Build history of the part. All positions in model axes, mm. Face numbers are marked on the shaded views. A direction names the side the tool comes from. Give positions to 0.01 mm unless a question says otherwise; leave off trailing zeros. Order: outer loops, then holes, each group sorted by start corner. A loop starts at its lowest first (then second) coordinate and runs counter-clockwise, first axis right, second up. Notation, with made-up numbers: (31.5, 89) - (79.5, 89) arc R26 ccw to (79.5, 117) - close; hole circle Ø5 at (58, 11). An arc over 180 degrees is marked (long way). Write each question's results on one line, items separated by ' | '. Start each with the question number.
1) Drill centre lines: line 1 along Y through (x, z) = (0, 2.4); line 2 along Z through (x, y) = (3, -6); line 3 along X through (y, z) = (-2.75, 16.5). Where is each one in solid material? Low to high. Write a range as from..to.
2) Cut at C-C on y = 0. List the corners of the cut face in (x, z).
3) Cut at D-D on y = 7.5. List the corners of the cut face in (x, z), plus the area to 3 significant figures.
4) Tool access for the marked faces 5 and 6: list every direction of +Z, -Z, +X, -X, +Y, -Y with a clear straight run to the whole face (end or side of a thin tool).
5) Drop flat-ended pins along their axis: pin 1 Ø12 at (y, z) = (-7, 11) entering from -X; pin 2 Ø10 at (x, y) = (0, 0) entering from -Z; pin 3 Ø1 at (y, z) = (-3.5, 5.5) entering from -X; pin 4 Ø6 at (y, z) = (0, 24) entering from -X. Give the stop position or say it passes through.
6) Two-plate mould, pull along Z, no slides. Class the marked faces 1, 2, 3 and 4: +Z half, -Z half, draft (parallel to the pull), parting line (faces both ways), or undercut.
7) Cut at A-A on x = -3. List the corners of the cut face in (y, z).
8) Cut at B-B on z = 24. List the corners of the cut face in (x, y).
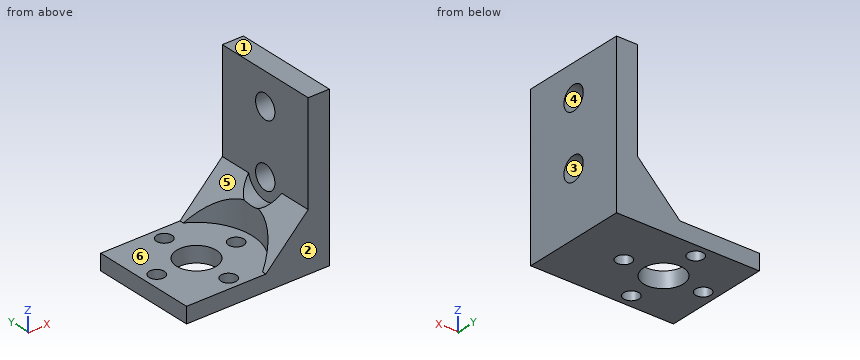
from build123d import *

# Parameters (mm, degrees)
SKETCH_1_W                   = 20
SKETCH_1_H                   = 20
EXTRUDE_1_DEPTH              = 3
SKETCH_8_W                   = 3
SKETCH_8_H                   = 20
EXTRUDE_3_DEPTH              = 3
SKETCH_2_R                   = 3.75
CUT_EXTRUDE_1_DEPTH          = 17.673332001
SKETCH_3_W                   = 4
SKETCH_3_H                   = 20
EXTRUDE_2_DEPTH              = 30
CHAMFER_1_SIZE               = 8
SKETCH_9_R                   = 10.5
CUT_EXTRUDE_2_DEPTH          = 27
HOLE_WIZARD_M4_1_D           = 4.5
HOLE_WIZARD_M4_1_CBORE_D     = 8
HOLE_WIZARD_M4_1_CBORE_DEPTH = 23
HOLE_WIZARD_M2_5_1_D         = 2.9


with BuildPart() as part:
    # 草圖1 → 填料-伸長1 (new body)
    with BuildSketch(Plane.XY):
        Rectangle(SKETCH_1_W, SKETCH_1_H)
    extrude(amount=EXTRUDE_1_DEPTH)

    # 草圖8 → 填料-伸長3 (add)
    with BuildSketch(Plane(origin=(10, 0, 0), x_dir=(0, 0, -1), z_dir=(1, 0, 0))):
        with Locations((-1.5, 0)):
            Rectangle(SKETCH_8_W, SKETCH_8_H)
    extrude(amount=EXTRUDE_3_DEPTH)

    # 草圖2 → 除料-伸長1 (cut, through all)
    with BuildSketch(Plane.XY.offset(3)):
        Circle(SKETCH_2_R)
    extrude(amount=-CUT_EXTRUDE_1_DEPTH, mode=Mode.SUBTRACT)

    # 草圖3 → 填料-伸長2 (add)
    with BuildSketch(Plane(origin=(0, 0, 0), x_dir=(-1, 0, 0), z_dir=(0, 0, -1))):
        with Locations((-15, 0)):
            Rectangle(SKETCH_3_W, SKETCH_3_H)
    extrude(amount=-EXTRUDE_2_DEPTH)

    # 導角1
    chamfer_1_edges = [part.edges().sort_by_distance(p)[0] for p in [
        (13, 0, 3),
    ]]
    chamfer(chamfer_1_edges, length=CHAMFER_1_SIZE)

    # 草圖9 → 除料-伸長2 (cut)
    with BuildSketch(Plane.XY.offset(30)):
        Circle(SKETCH_9_R)
    extrude(amount=-CUT_EXTRUDE_2_DEPTH, mode=Mode.SUBTRACT)

    # M4 凹頭蓋螺釘的柱孔1 (through all)
    with Locations(Plane.ZY.offset(10)):
        with Locations((24, 0), (12, 0)):
            CounterBoreHole(HOLE_WIZARD_M4_1_D / 2, HOLE_WIZARD_M4_1_CBORE_D / 2, HOLE_WIZARD_M4_1_CBORE_DEPTH)

    # M2.5 餘隙孔1 (through all)
    with Locations(Plane(origin=(0, 0, 0), x_dir=(-1, 0, 0), z_dir=(0, 0, -1))):
        with Locations((0, -7.5), (0, 7.5), (-7.5, 0), (7.5, 0)):
            Hole(HOLE_WIZARD_M2_5_1_D / 2)


solid = part.part
Results:
1) line 1: -10..-8.95, -6.05..-3.75, 3.75..6.05, 8.95..10 | line 2: 0..3 | line 3: 13..17
2) outline: (-10, 0) - (-8.95, 0) - (-8.95, 3) - (-10, 3) - close; (-6.05, 0) - (-3.75, 0) - (-3.75, 3) - (-6.05, 3) - close; (3.75, 0) - (6.05, 0) - (6.05, 3) - (3.75, 3) - close; (8.95, 0) - (17, 0) - (17, 9.75) - (13, 9.75) - (13, 8) - (10.5, 8) - (10.5, 3) - (8.95, 3) - close; (13, 14.25) - (17, 14.25) - (17, 21.75) - (13, 21.75) - close; (13, 26.25) - (17, 26.25) - (17, 30) - (13, 30) - close
3) outline: (-10, 0) - (-1.45, 0) - (-1.45, 3) - (-10, 3) - close; (1.45, 0) - (17, 0) - (17, 30) - (13, 30) - (13, 11) - (7.35, 5.35) - (7.35, 3) - (1.45, 3) - close | area: 210 mm^2
4) face 5: +Z, -X, +Y, -Y | face 6: +Z, -X
5) pin 1: x = 7.05 | pin 2: z = 0 | pin 3: x = 9.71 | pin 4: x = 13
6) face 1: +Z half | face 2: draft | face 3: undercut | face 4: undercut
7) outline: (-10, 0) - (-2.25, 0) - (-2.25, 3) - (-10, 3) - close; (2.25, 0) - (10, 0) - (10, 3) - (2.25, 3) - close
8) outline: (13, -10) - (17, -10) - (17, -2.25) - (13, -2.25) - close; (13, 2.25) - (17, 2.25) - (17, 10) - (13, 10) - close
